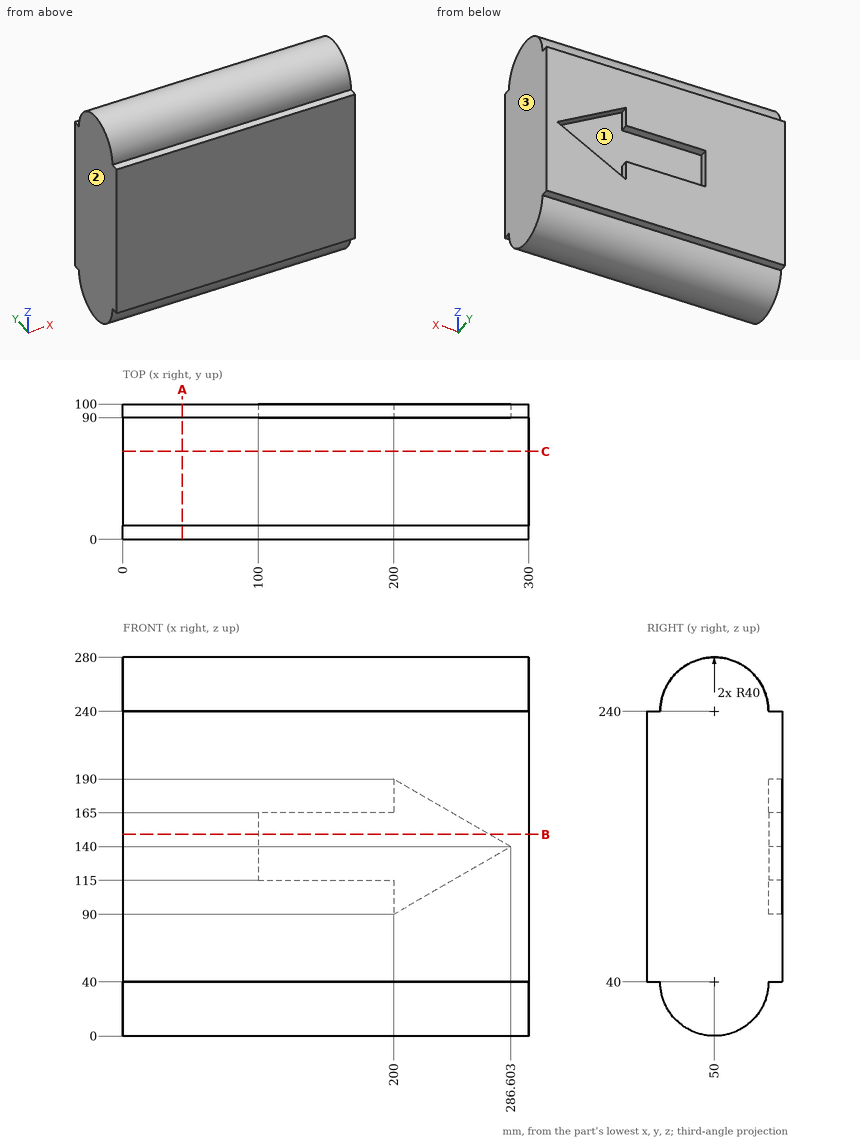
Answer from the drawing. Dimensions are ordinates in mm from the lowest x, y and z of the part. Round coordinates to 2 decimals unless told otherwise and drop trailing zeros. Loops run counter-clockwise (first coordinate to the right, second up) from the corner with the lowest first, then second, coordinate; pieces in that order, holes last. Notation, with made-up numbers: (-39, -37) - (-24, -37) arc R32 cw to (-24, -8) - close; hole circle Ø7 at (-22, 55). An arc over 180 degrees is marked (long way). One line per item, written item: value.
Q1. Each of these flat-tipped pins is pushed along its axis until it touches: pin 1 Ø4 at (x, z) = (222.5, 32.5) entering from -Y; pin 2 Ø3 at (x, y) = (209.5, 68.5) entering from -Z; pin 3 Ø10 at (x, y) = (105.5, 39) entering from +Z. Where does it stop, or does it pass through?
Check values:
pin 1: y = 10.38
pin 2: z = 3.79
pin 3: z = 279.55
Q2. Find section B-B on z = 149. Give the vertices of the cut face in (x, y) (1 decimal).
Check values:
outline: (0, 0) - (300, 0) - (300, 100) - (271, 100) - (271, 90) - (100, 90) - (100, 100) - (0, 100) - close
Q3. Straight lines are drawn through the part: probe 1 along Y at (x, z) = (200.5, 111.5); probe 2 along Z at (x, y) = (49, 52); probe 3 along Z at (x, y) = (287, 28.5). For each, find the intervals that lie inside material, in ascending order.
Check values:
probe 1: 0 to 90
probe 2: 0.05 to 279.95
probe 3: 6.27 to 273.73
Q4. Find section C-C on y = 65. Give the vertices of the cut face in (x, z), and give its area (3 significant figures).
Check values:
outline: (0, 2.92) - (300, 2.92) - (300, 277.08) - (0, 277.08) - close
area: 82,200 mm2
Q5. The mould has two halves that part along X. Classify the marked faces 1, 2 and 3: +X half, -X half, draft (parallel to the pull), parting line (faces both ways), or undercut.
Check values:
face 1: undercut
face 2: -X half
face 3: +X half
Q6. Find section A-A on x = 44. Give the vertices of the cut face in (y, z).
Check values:
outline: (0, 40) - (10, 40) arc R40 ccw to (90, 40) - (100, 40) - (100, 240) - (90, 240) arc R40 ccw to (10, 240) - (0, 240) - close
